```python
from build123d import *

# Parameters (mm, degrees)
SKETCH1_R           = 36.5
SKETCH1_R_2         = 34.5
BOSS_EXTRUDE1_DEPTH = 140
SKETCH3_W           = 6.5
SKETCH3_H           = 120
CUT_EXTRUDE1_DEPTH  = 150.212935096
CIRPATTERN1_COUNT   = 2
CIRPATTERN1_ANGLE   = 90
SKETCH4_R           = 2
CUT_EXTRUDE2_DEPTH  = 150.212935096


with BuildPart() as part:
    # Sketch1 → Boss-Extrude1 (new body)
    with BuildSketch(Plane(origin=(0, 0, 0), x_dir=(1, 0, 0), z_dir=(0, 1, 0))):
        with Locations(Location((0, 0, 0), (0, 0, 270))):
            Circle(SKETCH1_R)
        with Locations(Location((0, 0, 0), (0, 0, 270))):
            Circle(SKETCH1_R_2, mode=Mode.SUBTRACT)
    extrude(amount=BOSS_EXTRUDE1_DEPTH)

    # Sketch3 → Cut-Extrude1 (cut, symmetric)
    with BuildSketch(Plane.XY):
        with Locations((0, 70)):
            Rectangle(SKETCH3_W, SKETCH3_H)
    cut_extrude1 = extrude(amount=CUT_EXTRUDE1_DEPTH, both=True, mode=Mode.SUBTRACT)

    # CirPattern1: Cut-Extrude1 ×2 about axis
    cirpattern1_axis = Axis((0, 125, 0), (0, -1, 0))
    for i in range(1, CIRPATTERN1_COUNT):
        add(cut_extrude1.rotate(cirpattern1_axis, i * CIRPATTERN1_ANGLE / (CIRPATTERN1_COUNT - 1)), mode=Mode.SUBTRACT)

    # Sketch4 → Cut-Extrude2 (cut, through all)
    with BuildSketch(Plane(origin=(0, 0, 0), x_dir=(0.7071067811865477, 0, 0.7071067811865475), z_dir=(-0.7071067811865475, 0, 0.7071067811865477))):
        with Locations(Location((0, 25, 0), (0, 0, 180))):
            Circle(SKETCH4_R)
    extrude(amount=CUT_EXTRUDE2_DEPTH, mode=Mode.SUBTRACT)


solid = part.part
```
Build history of the part. All positions in model axes, mm. Give positions to 0.01 mm unless a question says otherwise; leave off trailing zeros. Loops run counter-clockwise (first coordinate to the right, second up) from the corner with the lowest first, then second, coordinate; pieces in that order, holes last.
Item 1: Pull direction Z, two halves, no side cores. Call faces 1 (the face through (-26.38, 25.77, 23.77)), 2 (the face through (10.964, 69.02, 34.814)), 3 (the face through (22, 0, 27)): released by +Z, released by -Z, zero draft, split by the parting line, or undercut.
Answers follow:
face 1: undercut
face 2: split by the parting line
face 3: zero draft
Item 2: Drill centre lines: line 1 (X direction, y = 54.5, z = -4); line 2 (Z direction, x = 6, y = 13); line 3 (X direction, y = 80, z = -14.5). Where is each one in solid material? Low to high.
Answers follow:
line 1: x = -36.28 to -34.27, 34.27 to 36.28
line 2: z = -36 to -33.97, 33.97 to 36
line 3: x = -33.5 to -31.3, 31.3 to 33.5
Item 3: Slice it at A-A, the plane y = 65.5. List the corners of the cut face in (x, z), and give its area (3 significant figures).
Answers follow:
outline: (-36.36, -3.25) arc R36.5 ccw to (-3.25, -36.36) - (-3.25, -34.35) arc R34.5 cw to (-34.35, -3.25) - close; (-36.36, 3.25) - (-34.35, 3.25) arc R34.5 cw to (-3.25, 34.35) - (-3.25, 36.36) arc R36.5 ccw to start; (3.25, -36.36) arc R36.5 ccw to (36.36, -3.25) - (34.35, -3.25) arc R34.5 cw to (3.25, -34.35) - close; (3.25, 34.35) arc R34.5 cw to (34.35, 3.25) - (36.36, 3.25) arc R36.5 ccw to (3.25, 36.36) - close
area: 394 mm2
Item 4: Slice it at C-C, the plane x = 22.5. List the corners of the cut face in (y, z), and give its area (3 significant figures).
Answers follow:
outline: (0, -28.74) - (140, -28.74) - (140, -26.15) - (0, -26.15) - close; (0, 26.15) - (140, 26.15) - (140, 28.74) - (0, 28.74) - close
area: 724 mm2
Item 5: Slice it at B-B, the plane z = 0. List the corners of the cut face in (x, y), and give its area (3 significant figures).
Answers follow:
outline: (-36.5, 0) - (-34.5, 0) - (-34.5, 10) - (-36.5, 10) - close; (-36.5, 130) - (-34.5, 130) - (-34.5, 140) - (-36.5, 140) - close; (34.5, 0) - (36.5, 0) - (36.5, 10) - (34.5, 10) - close; (34.5, 130) - (36.5, 130) - (36.5, 140) - (34.5, 140) - close
area: 80.0 mm2
Item 6: Slice it at D-D, the plane z = 12. List the corners of the cut face in (x, y).
Answers follow:
outline: (-34.47, 0) - (-32.35, 0) - (-32.35, 140) - (-34.47, 140) - close; (32.35, 0) - (34.47, 0) - (34.47, 140) - (32.35, 140) - close
Item 7: Flat gauge pins, fed straight in: pin 1 (6 mm diameter, centred on x = 3.5, y = 117, fed in from -Z) (3 decimals); pin 2 (3 mm diameter, centred on y = 109.5, z = -24.5, fed in from +X); pin 3 (5 mm diameter, centred on y = 23.5, z = -13, fed in from -X). Where does each tip first touch, or does it go through?
Answers follow:
pin 1: stops at z = -36.355
pin 2: stops at x = 28.34
pin 3: stops at x = -34.96
